For this review, take the finished solid that the model builds, in its own axes (mm). A direction names the side the tool comes from. Give positions to 0.01 mm unless a question says otherwise; leave off trailing zeros. One line per question, with ' | ' between items. Start each with the question number.
(1) Wall thickness on probe 1 along Y at (x, z) = (0, -124.5); probe 2 along X at (y, z) = (10, -266.5); probe 3 along Y at (x, z) = (-5.25, -278): over which ranges is each line inside the solid? List them lowest first.
(2) Insertion check: P1, Ø0.7, axis at y = -11, z = -210.5, coming from the -X side; P2, Ø1.2, axis at y = -8.5, z = -182, coming from the +X side; P3, Ø1.5, axis at x = -2, z = -267, coming from the +Y side. Each pin has a flat end and moves straight along its axis. Give the tip position at first contact, or say it passes through.
(3) Draft analysis for pull direction Y (two halves, no side actions). For faces 3 (the flat face through (6, -20, -187)), 4 (the flat face through (0, 6, -187)), 5 (the flat face through (10, -16, -187)), state which applies: +Y half, -Y half, draft (parallel to the pull), parting line (faces both ways), or undercut.
(4) Tool access review of faces 1 (the flat face through (0, -6, -187)), 2 (the flat face through (-6, -20, -187)): name each direction out of +Z, -Z, +X, -X, +Y, -Y from which nothing blocks a thin tool from reaching the whole face with its end or side.
(5) Consider section A-A (z = -194). Give the number of separate pieces and of enclosed holes in the cut face, and give its area (3 significant figures).
Autodesk Inventor part; units mm, degrees
ref_plane "C1_XY" through (0, 0, 0) normal (0, 0, 1) x (1, 0, 0)
ref_plane "C1_YZ" through (0, 0, 0) normal (1, 0, 0) x (0, 1, 0)
ref_plane "C1_ZX" through (0, 0, 0) normal (0, 1, 0) x (0, 0, 1)
sketch "Sketch_1" plane through (0, 0, 0) normal (0, 0, 1) x (1, 0, 0)
  line L0 (-10, -7) -> (-8, -7)
  line L1 (-8, -7) -> (-8, -4)
  line L2 (-8, -4) -> (-7.0607, -4)
  line L3 (-7.0607, -4) -> (-4, -7.0607)
  line L4 (-4, -7.0607) -> (-4, -9.4804)
  line L5 (-4, -9.4804) -> (-3.7, -10)
  line L6 (-3.7, -10) -> (-4, -10.5196)
  line L7 (-4, -10.5196) -> (-4, -12.9393)
  line L8 (-4, -12.9393) -> (-7.0607, -16)
  line L9 (-7.0607, -16) -> (-8, -16)
  line L10 (-8, -16) -> (-8, -13)
  line L11 (-8, -13) -> (-10, -13)
  line L12 (-10, -13) -> (-10, -19)
  arc A0 (-10, -19) -> (-9, -20) centre (-9, -19) ccw
  line L13 (-9, -20) -> (-3, -20)
  line L14 (-3, -20) -> (-3, -18)
  line L15 (-3, -18) -> (-6, -18)
  line L16 (-6, -18) -> (-6, -17.0607)
  line L17 (-6, -17.0607) -> (-2.9393, -14)
  line L18 (-2.9393, -14) -> (-0.5196, -14)
  line L19 (-0.5196, -14) -> (0, -13.7)
  line L20 (0, -13.7) -> (0.5196, -14)
  line L21 (0.5196, -14) -> (2.9393, -14)
  line L22 (2.9393, -14) -> (6, -17.0607)
  line L23 (6, -17.0607) -> (6, -18)
  line L24 (6, -18) -> (3, -18)
  line L25 (3, -18) -> (3, -20)
  line L26 (3, -20) -> (9, -20)
  arc A1 (9, -20) -> (10, -19) centre (9, -19) ccw
  line L27 (10, -19) -> (10, -13)
  line L28 (10, -13) -> (8, -13)
  line L29 (8, -13) -> (8, -16)
  line L30 (8, -16) -> (7.0607, -16)
  line L31 (7.0607, -16) -> (4, -12.9393)
  line L32 (4, -12.9393) -> (4, -10.5196)
  line L33 (4, -10.5196) -> (3.7, -10)
  line L34 (3.7, -10) -> (4, -9.4804)
  line L35 (4, -9.4804) -> (4, -7.0607)
  line L36 (4, -7.0607) -> (7.0607, -4)
  line L37 (7.0607, -4) -> (8, -4)
  line L38 (8, -4) -> (8, -7)
  line L39 (8, -7) -> (10, -7)
  line L40 (10, -7) -> (10, 7)
  line L41 (10, 7) -> (8, 7)
  line L42 (8, 7) -> (8, 4)
  line L43 (8, 4) -> (7.0607, 4)
  line L44 (7.0607, 4) -> (4, 7.0607)
  line L45 (4, 7.0607) -> (4, 9.4804)
  line L46 (4, 9.4804) -> (3.7, 10)
  line L47 (3.7, 10) -> (4, 10.5196)
  line L48 (4, 10.5196) -> (4, 12.9393)
  line L49 (4, 12.9393) -> (7.0607, 16)
  line L50 (7.0607, 16) -> (8, 16)
  line L51 (8, 16) -> (8, 13)
  line L52 (8, 13) -> (10, 13)
  line L53 (10, 13) -> (10, 19)
  arc A2 (10, 19) -> (9, 20) centre (9, 19) ccw
  line L54 (9, 20) -> (3, 20)
  line L55 (3, 20) -> (3, 18)
  line L56 (3, 18) -> (6, 18)
  line L57 (6, 18) -> (6, 17.0607)
  line L58 (6, 17.0607) -> (2.9393, 14)
  line L59 (2.9393, 14) -> (0.5196, 14)
  line L60 (0.5196, 14) -> (0, 13.7)
  line L61 (0, 13.7) -> (-0.5196, 14)
  line L62 (-0.5196, 14) -> (-2.9393, 14)
  line L63 (-2.9393, 14) -> (-6, 17.0607)
  line L64 (-6, 17.0607) -> (-6, 18)
  line L65 (-6, 18) -> (-3, 18)
  line L66 (-3, 18) -> (-3, 20)
  line L67 (-3, 20) -> (-9, 20)
  arc A3 (-9, 20) -> (-10, 19) centre (-9, 19) ccw
  line L68 (-10, 19) -> (-10, 13)
  line L69 (-10, 13) -> (-8, 13)
  line L70 (-8, 13) -> (-8, 16)
  line L71 (-8, 16) -> (-7.0607, 16)
  line L72 (-7.0607, 16) -> (-4, 12.9393)
  line L73 (-4, 12.9393) -> (-4, 10.5196)
  line L74 (-4, 10.5196) -> (-3.7, 10)
  line L75 (-3.7, 10) -> (-4, 9.4804)
  line L76 (-4, 9.4804) -> (-4, 7.0607)
  line L77 (-4, 7.0607) -> (-7.0607, 4)
  line L78 (-7.0607, 4) -> (-8, 4)
  line L79 (-8, 4) -> (-8, 7)
  line L80 (-8, 7) -> (-10, 7)
  line L81 (-10, 7) -> (-10, -7)
  line L82 (-8, 1.7) -> (-8, -1.7)
  arc A4 (-8, -1.7) -> (-7.7, -2) centre (-7.7, -1.7) ccw
  line L83 (-7.7, -2) -> (-7.0636, -2)
  arc A5 (-6.8515, -2.0879) -> (-7.0636, -2) centre (-7.0636, -2.3) ccw
  line L84 (-6.8515, -2.0879) -> (-2.9393, -6)
  line L85 (-2.9393, -6) -> (2.9393, -6)
  line L86 (2.9393, -6) -> (6.8515, -2.0879)
  arc A6 (7.0636, -2) -> (6.8515, -2.0879) centre (7.0636, -2.3) ccw
  line L87 (7.0636, -2) -> (7.7, -2)
  arc A7 (7.7, -2) -> (8, -1.7) centre (7.7, -1.7) ccw
  line L88 (8, -1.7) -> (8, 1.7)
  arc A8 (8, 1.7) -> (7.7, 2) centre (7.7, 1.7) ccw
  line L89 (7.7, 2) -> (7.0636, 2)
  arc A9 (6.8515, 2.0879) -> (7.0636, 2) centre (7.0636, 2.3) ccw
  line L90 (6.8515, 2.0879) -> (2.9393, 6)
  line L91 (2.9393, 6) -> (-2.9393, 6)
  line L92 (-2.9393, 6) -> (-6.8515, 2.0879)
  arc A10 (-7.0636, 2) -> (-6.8515, 2.0879) centre (-7.0636, 2.3) ccw
  line L93 (-7.0636, 2) -> (-7.7, 2)
  arc A11 (-7.7, 2) -> (-8, 1.7) centre (-7.7, 1.7) ccw
extrude "Extrusion1" add sketch "Sketch_1" against normal blind 380
sketch "Sketch2" plane through (0, 0, -380) normal (0, 0, -1) x (-1, 0, 0)
  point P0 (0, 10)
hole "Hole1" at (0, 10, -380) direction (0, 0, 1) diameter 4.2 depth 380
pattern_linear "Rectangular Pattern1" count 2 spacing 20 along (0, -1, 0) of "Hole1"
ref_plane "C1_XY" through (0, 0, 0) normal (0, 0, 1) x (1, 0, 0)
ref_plane "C1_YZ" through (0, 0, 0) normal (1, 0, 0) x (0, 1, 0)
ref_plane "C1_ZX" through (0, 0, 0) normal (0, 1, 0) x (0, 0, 1)
properties part number "HFS5-2040-380"
A:
1) probe 1: y = -13.7 to -12.1, -7.9 to -6, 6 to 7.9, 12.1 to 13.7 | probe 2: x = -3.7 to -2.1, 2.1 to 3.7 | probe 3: y = -20 to -18, -16.31 to -14.19, -5.81 to -3.69, 3.69 to 5.81, 14.19 to 16.31, 18 to 20
2) P1: stops at x = -4 | P2: stops at x = 4 | P3: stops at y = 14
3) face 3: -Y half | face 4: undercut | face 5: draft
4) face 1: +Z, -Z | face 2: +Z, -Z, +X, -X, -Y
5) separate pieces: 1 | enclosed holes: 3 | area: 324 mm^2
